```python
from build123d import *

# Parameters (mm, degrees)
F0_W     = 19.9
F0_H     = 40.7
F1_DEPTH = 41
F3_W     = 19.9
F3_H     = 7
F3_R     = 2
F4_DEPTH = 3
F5_R     = 4
F6_DEPTH = 4


with BuildPart() as f1:
    # F0 (on Top) → F1 (new body)
    with BuildSketch(Plane.XY):
        with Locations((0, -10.75)):
            Rectangle(F0_W, F0_H)
    extrude(amount=F1_DEPTH)

    # F3 (on offset) → F4 (join)
    with BuildSketch(Plane.XY.offset(29)):
        with Locations((0, 13.1)):
            Rectangle(F3_W, F3_H)
        with Locations((-4.75, 13.6)):
            Circle(F3_R, mode=Mode.SUBTRACT)
        with Locations((4.75, 13.6)):
            Circle(F3_R, mode=Mode.SUBTRACT)
        with Locations((0, -34.6)):
            Rectangle(F3_W, F3_H)
        with Locations((-4.75, -35.1)):
            Circle(F3_R, mode=Mode.SUBTRACT)
        with Locations((4.75, -35.1)):
            Circle(F3_R, mode=Mode.SUBTRACT)
    extrude(amount=F4_DEPTH)

    # F5 (on face) → F6 (join)
    with BuildSketch(Plane.XY.offset(41)):
        Circle(F5_R)
    extrude(amount=F6_DEPTH)


solid = f1.part
```
Geometry: final body of the model. Coordinates: model frame, mm. A direction names the side the tool comes from. Round coordinates to 2 decimals unless told otherwise and drop trailing zeros. Write each loop counter-clockwise with the first axis right and the second up, starting at its lowest first coordinate (ties: lowest second). Pieces come first, ordered by that corner, then holes. Notation, with made-up numbers: (80.25, -38) -> (97.25, -38) arc R26 ccw to (97.25, -22) -> close; hole circle Ø11 at (37.5, 85.25). An arc over 180 degrees is marked (long way). Use CSV: the item, a comma, the result in double quotes. Start each with the question number.
Q1. Section A-A (x = 4.75). Return loops of the section in (y, z).
Q2. Reachability of faces 4 (the face through (0, -35, 32)), 5 (the face through (0, 13, 29)), 6 (the face through (0, -31.1, 14)), 7 (the face through (0, 9.6, 36)), 8 (the face through (-0.867, -3.905, 42.972)) from +Z, -Z, +X, -X, +Y, -Y: full face, straight path, thin tool, end or side. Return the list, or none.
Q3. Line query: L1, parallel to Y at x = 4.75, z = 30; L2, parallel to X at y = -35, z = 30; L3, parallel to Z at x = 4, y = -18. Output: solid intervals per line, ascending.
Q4. Section D-D (y = 0). Return loops of the section in (x, z), plus the area to 3 significant figures.
Q5. First-contact query: pin 1 Ø10 at (x, y) = (-2.5, -20) entering from +Z; pin 2 Ø1 at (x, y) = (6.5, -32.5) entering from +Z; pin 3 Ø2.5 at (x, z) = (-2, 38) entering from +Y. Flat tips, straight axial feed; report the tip coordinate or a pass-through.
Q6. Pull-direction query (X, two-part tool) for faces 1 (the face through (-9.95, -11, 20)), 2 (the face through (-3.827, -36.874, 30.479)), 3 (the face through (0, 0, 45)); classes: pulls with the +X half, pulls with the -X half, needs draft (parallel to the pull), parting line crosses it, or undercut.
Q7. Section C-C (z = 30). Return loops of the section in (x, y), plus the area to 3 significant figures.
Q8. Section B-B (y = -35.1). Return loops of the section in (x, z).
Result sheet:
1,outline,"(-38.1, 29) -> (-37.1, 29) -> (-37.1, 32) -> (-38.1, 32) -> close; (-33.1, 29) -> (-31.1, 29) -> (-31.1, 0) -> (9.6, 0) -> (9.6, 29) -> (11.6, 29) -> (11.6, 32) -> (9.6, 32) -> (9.6, 41) -> (-31.1, 41) -> (-31.1, 32) -> (-33.1, 32) -> close; (15.6, 29) -> (16.6, 29) -> (16.6, 32) -> (15.6, 32) -> close"
2,face 4,"+Z, +X, -X, -Y"
2,face 5,"-Z, +X, -X, +Y"
2,face 6,"-Z, +X, -X, -Y"
2,face 7,"+Z, +X, -X, +Y"
2,face 8,"+Z"
3,L1,"-38.1 to -37.1, -33.1 to 11.6, 15.6 to 16.6"
3,L2,"-9.95 to -6.75, -2.75 to 2.75, 6.75 to 9.95"
3,L3,"0 to 41"
4,outline,"(-9.95, 0) -> (9.95, 0) -> (9.95, 41) -> (4, 41) -> (4, 45) -> (-4, 45) -> (-4, 41) -> (-9.95, 41) -> close"
4,area,"848 mm²"
5,pin 1,"z = 41"
5,pin 2,"z = 32"
5,pin 3,"y = 9.6"
6,face 1,"pulls with the -X half"
6,face 2,"undercut"
6,face 3,"needs draft"
7,outline,"(-9.95, -38.1) -> (9.95, -38.1) -> (9.95, 16.6) -> (-9.95, 16.6) -> close; hole circle Ø4 at (-4.75, -35.1); hole circle Ø4 at (-4.75, 13.6); hole circle Ø4 at (4.75, -35.1); hole circle Ø4 at (4.75, 13.6)"
7,area,"1,040 mm²"
8,outline,"(-9.95, 29) -> (-6.75, 29) -> (-6.75, 32) -> (-9.95, 32) -> close; (-2.75, 29) -> (2.75, 29) -> (2.75, 32) -> (-2.75, 32) -> close; (6.75, 29) -> (9.95, 29) -> (9.95, 32) -> (6.75, 32) -> close"
